Could you check a few things on this model? Use its own coordinates, in mm. A direction names the side the tool comes from. Round coordinates to 2 decimals unless told otherwise and drop trailing zeros. Write each loop counter-clockwise with the first axis right and the second up, starting at its lowest first coordinate (ties: lowest second). Pieces come first, ordered by that corner, then holes. Notation, with made-up numbers: (9.25, 33) - (62.25, 33) arc R4 ccw to (62.25, 38) - close; hole circle Ø3 at (7, 54). An arc over 180 degrees is marked (long way). Write each question's results on one line, items separated by ' | '. Start each with the question number.
(1) Imagine slicing it at A-A on x = 0. Write out the boundary of the cut face in (y, z), then the cut area to 3 significant figures.
(2) Imagine slicing it at D-D on z = 30.5. Write out the boundary of the cut face in (x, y).
(3) Imagine slicing it at B-B on z = -43. Write out the boundary of the cut face in (x, y).
(4) On a 3-axis mill with a long thin cutter (end or side, diameter ignored), from which of +Z, -Z, +X, -X, +Y, -Y can I reach the whole of each face in a straight line? I mean faces 1 (the flat face through (0, -264.16, -23)), 2 (the cylindrical face through (1.536, -130.231, 11.226)). Say none if no direction works.
(5) Please list where these lines run through material, in increasing order: line 1 (Y direction, x = 48.5, z = 11); line 2 (Z direction, x = 2.5, y = -8.5); line 3 (X direction, y = -110.5, z = -26). Write a range as [from, to].
(6) For P1, Ø4, axis at x = 3.5, z = 28, coming from the -Y side; P2, Ø2, axis at x = -8.5, y = -18, coming from the -Z side; P3, Ø6, axis at x = -17.5, y = -79, coming from the +Z side, each with a flat end and sliding along its axis, tell me the tip position at first contact or that it passes through.
(7) Imagine slicing it at C-C on y = -191.5. Write out the boundary of the cut face in (x, z) (3 decimals), then the cut area to 3 significant figures.
```python
from build123d import *

# Parameters (mm, degrees)
SKETCH1_W      = 123.698
SKETCH1_H      = 142.748
EXTRUDE1_DEPTH = 207.518
SKETCH2_R      = 34.925
EXTRUDE2_DEPTH = 264.16


with BuildPart() as part:
    # Sketch1 → Extrude1 (new body)
    with BuildSketch(Plane(origin=(0, 0, 0), x_dir=(1, 0, 0), z_dir=(0, 1, 0))):
        with Locations((10.507234487, 23.665651739)):
            Rectangle(SKETCH1_W, SKETCH1_H)
    extrude(amount=EXTRUDE1_DEPTH)

    # Sketch2 → Extrude2 (add)
    with BuildSketch(Plane.XZ):
        with Locations(Location((0, -23.665651739, 0), (0, 0, 270))):
            Circle(SKETCH2_R)
    extrude(amount=EXTRUDE2_DEPTH)


solid = part.part
```
Response:
1) outline: (-264.16, -58.59) - (0, -58.59) - (0, -95.04) - (207.52, -95.04) - (207.52, 47.71) - (0, 47.71) - (0, 11.26) - (-264.16, 11.26) - close | area: 48,100 mm²
2) outline: (-51.34, 0) - (72.36, 0) - (72.36, 207.52) - (-51.34, 207.52) - close
3) outline: (-51.34, 0) - (-29.09, 0) - (-29.09, -264.16) - (29.09, -264.16) - (29.09, 0) - (72.36, 0) - (72.36, 207.52) - (-51.34, 207.52) - close
4) face 1: +Z, -Z, +X, -X, -Y | face 2: -Y
5) line 1: [0, 207.52] | line 2: [-58.5, 11.17] | line 3: [-34.85, 34.85]
6) P1: y = 0 | P2: z = -57.78 | P3: z = 8.11
7) outline: circle Ø69.85 at (0, -23.666) | area: 3,830 mm²
